```python
from build123d import *

# Parameters (mm, degrees)
BOSS_EXTRUDE1_DEPTH = 98.298
SKETCH2_W           = 98.298
SKETCH2_H           = 4.0005
BOSS_EXTRUDE2_DEPTH = 0.635


with BuildPart() as part:
    # Sketch1 → Boss-Extrude1 (new body)
    with BuildSketch(Plane(origin=(0, 0, 0), x_dir=(0, 0, -1), z_dir=(1, 0, 0))):
        with BuildLine():
            Line((-16.7005, 0), (-12.7, 0))
            ThreePointArc((-12.7, 0), (-4.860079591, 11.733270063), (8.980256121, 8.980256121))
            Line((8.980256121, 8.980256121), (11.809036799, 11.809036799))
            ThreePointArc((11.809036799, 11.809036799), (-6.391004662, 15.429250133), (-16.7005, 0))
        make_face()
    extrude(amount=BOSS_EXTRUDE1_DEPTH)

    # Sketch2 → Boss-Extrude2 (add)
    with BuildSketch(Plane.XZ):
        with Locations((49.149, 14.70025)):
            Rectangle(SKETCH2_W, SKETCH2_H)
    extrude(amount=BOSS_EXTRUDE2_DEPTH)


solid = part.part
```
Geometry: final body of the model. Coordinates: model frame, mm. Coordinates: 2 decimals unless noted, no trailing zeros. Loops run counter-clockwise (first coordinate to the right, second up) from the corner with the lowest first, then second, coordinate; pieces in that order, holes last. Notation, with made-up numbers: M 28.25,60 L 80.25,60 A13 cw 80.25,73 Z; hole C -32.5,47 d9. An arc over 180 degrees is marked long. Put each result on its own line as item: value.
(1) Material intervals for probe 1 along Z at (x, y) = (51, 10.5); probe 2 along Z at (x, y) = (48, 10.75); probe 3 along Y at (x, z) = (30, -7.5), sorted ascending.
Answer sheet:
probe 1: z = -10.5 to -7.14, 7.14 to 12.99
probe 2: z = -10.75 to -6.76, 6.76 to 12.78
probe 3: y = 10.25 to 14.92
(2) Cut plane C-C on y = 4.5. Return the cut outline in (x, z), then the cut area to 3 significant figures.
Answer sheet:
outline: M 0,11.88 L 98.3,11.88 L 98.3,16.08 L 0,16.08 Z
area: 414 mm^2
(3) First-contact query: pin 1 (4 mm diameter, centred on x = 11.5, y = 3.5, fed in from +Z); pin 2 (4 mm diameter, centred on x = 58, z = -5, fed in from +Y); pin 3 (1.5 mm diameter, centred on x = 84, y = 14, fed in from -Z). Flat tips, straight axial feed; report the tip coordinate or a pass-through.
Answer sheet:
pin 1: stops at z = 16.63
pin 2: stops at y = 16.43
pin 3: stops at z = -10.17
(4) Cut plane A-A on x = 44. Return the cut outline in (y, z) (1 decimal).
Answer sheet:
outline: M -0.6,12.7 L 0,12.7 A12.7 cw 9,-9 L 11.8,-11.8 A16.7 ccw 0,16.7 L -0.6,16.7 Z
(5) Cut plane B-B on z = 6.5. Return the cut outline in (x, y).
Answer sheet:
outline: M 0,10.91 L 98.3,10.91 L 98.3,15.38 L 0,15.38 Z
